The listing builds one solid part. Answer for the finished solid, in the listing's coordinates (mm). Face numbers are marked on the shaded views. Coordinates: 2 decimals unless noted, no trailing zeros. Order: outer loops, then holes, each group sorted by start corner. A loop starts at its lowest first (then second) coordinate and runs counter-clockwise, first axis right, second up. Notation, with made-up numbers: (48.25, 46.5) - (75.25, 46.5) arc R16 cw to (75.25, 62.5) - close; hole circle Ø3 at (55.5, -32). An arc over 180 degrees is marked (long way). One line per item, written item: value. Start each with the question number.
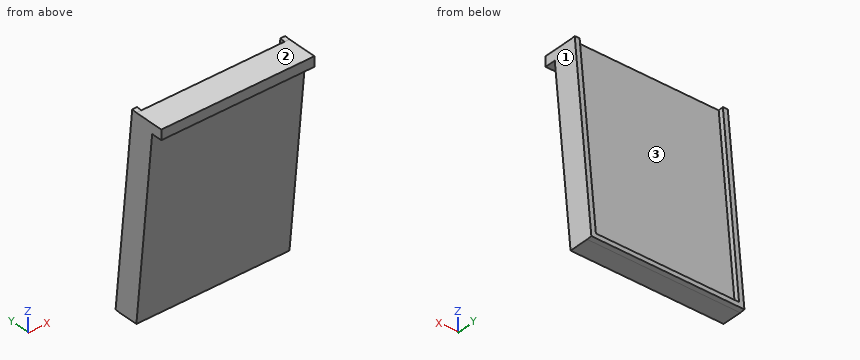
```python
from build123d import *

# Parameters (mm, degrees)
BOSS_EXTRUDE1_DEPTH = 155
SKETCH7_W           = 155
SKETCH7_H           = 20
BOSS_EXTRUDE4_DEPTH = 10
SKETCH8_W           = 145
SKETCH8_H           = 5
BOSS_EXTRUDE5_DEPTH = 5


with BuildPart() as part:
    # Sketch4 → Boss-Extrude1 (new body)
    with BuildSketch(Plane(origin=(0, 0, 0), x_dir=(0, 0, -1), z_dir=(1, 0, 0))):
        Polygon((0, 0), (0, 20), (198.997487421, 40), (198.997487421, 20), align=None)
    extrude(amount=BOSS_EXTRUDE1_DEPTH)

    # Sketch7 → Boss-Extrude4 (add)
    with BuildSketch(Plane.XY):
        with Locations((77.5, 0)):
            Rectangle(SKETCH7_W, SKETCH7_H)
    extrude(amount=-BOSS_EXTRUDE4_DEPTH)

    # Sketch8 → Boss-Extrude5 (add)
    with BuildSketch(Plane(origin=(0, 19.8, 1.989974874), x_dir=(1, 0, 0), z_dir=(0, 0.994987437, 0.1))):
        Polygon((5, 202), (0, 202), (0, 2), (5, 2), (5, 197), align=None)
        with Locations((77.5, 199.5)):
            Rectangle(SKETCH8_W, SKETCH8_H)
        Polygon((155, 202), (150, 202), (150, 197), (150, 2), (155, 2), align=None)
    extrude(amount=BOSS_EXTRUDE5_DEPTH)


solid = part.part
```
(1) The part is cut by section C-C on y = 17. Determine the outline of the cut face in (x, z).
(2) Flat-ended cylindrical pins translate along their axes: pin 1 Ø1.5 at (x, y) = (33, -2.5) entering from -Z; pin 2 Ø8 at (x, z) = (18.5, -47) entering from -Y; pin 3 Ø6 at (y, z) = (26, -107) entering from -X; pin 4 Ø1 at (x, y) = (88.5, -0.5) entering from +Z. Find the tip coordinate at first contact, or state that the pin passes through.
(3) The part is cut by section B-B on z = -106. Determine the outline of the cut face in (x, y).
(4) Consider probe 1 along Y at (x, z) = (42, -119.5); probe 2 along Y at (x, z) = (44.5, -59.5); probe 3 along Z at (x, y) = (25, 42.5). Determine where each line is inside the solid, lowest interval first.
(5) The part is cut by section A-A on x = 13.5. Determine the outline of the cut face in (y, z).
(6) For a pull along X with two mould halves and no side action, classify the marked faces 1, 2 and 3 as pulls with the +X half, pulls with the -X half, needs draft (parallel to the pull), parting line crosses it, or undercut.
Completed:
1. outline: (0, -169.15) - (155, -169.15) - (155, 0) - (0, 0) - close
2. pin 1: stops at z = -10
2. pin 2: stops at y = 4.32
2. pin 3: stops at x = 0
2. pin 4: stops at z = 0
3. outline: (0, 10.65) - (155, 10.65) - (155, 35.68) - (150, 35.68) - (150, 30.65) - (5, 30.65) - (5, 35.68) - (0, 35.68) - close
4. probe 1: y = 12.01 to 32.01
4. probe 2: y = 5.98 to 25.98
4. probe 3: z = -198.75 to -193.72
5. outline: (-10, -10) - (1.01, -10) - (20, -199) - (40, -199) - (44.97, -198.5) - (44.47, -193.52) - (39.5, -194.02) - (20, 0) - (-10, 0) - close
6. face 1: pulls with the +X half
6. face 2: needs draft
6. face 3: undercut
